```python
from build123d import *

# Parameters (mm, degrees)
EXTRUDE_1_DEPTH     = 25
EXTRUDE_2_DEPTH     = 2
CUT_EXTRUDE_1_DEPTH = 15
SKETCH_4_R          = 1.15
EXTRUDE_3_DEPTH     = 15
SKETCH_5_W          = 6.2
SKETCH_5_H          = 22
CUT_EXTRUDE_2_DEPTH = 74.581891949
SKETCH_6_W          = 6.2
SKETCH_6_H          = 2
CUT_EXTRUDE_3_DEPTH = 74.581891949
EXTRUDE_4_DEPTH     = 12
EXTRUDE_5_DEPTH     = 12


with BuildPart() as part:
    # 草图1 → 凸台-拉伸1 (new body)
    with BuildSketch(Plane.XY):
        Polygon((19.5, 14.714466094), (19.5, -3.035533906), (24.5, -3.035533906), (31.571067812, 4.035533906), (31.571067812, 41.75), (21.571067812, 51.75), (-21.571067812, 51.75), (-31.571067812, 41.75), (-31.571067812, 4.035533906), (-24.5, -3.035533906), (-19.5, -3.035533906), (-19.5, 14.714466094), (-26.571067812, 21.785533906), (-26.571067812, 36.75), (-21.571067812, 41.75), (21.571067812, 41.75), (26.571067812, 36.75), (26.571067812, 21.785533906), align=None)
    extrude(amount=EXTRUDE_1_DEPTH)

    # 草图2 → 凸台-拉伸2 (add)
    with BuildSketch(Plane.XY.offset(25)):
        Polygon((-26.571067812, 30.27081528), (-19.5, 23.199747468), (-19.5, 14.714466094), (-26.571067812, 21.785533906), align=None)
        Polygon((26.571067812, 30.27081528), (19.5, 23.199747468), (19.5, 14.714466094), (26.571067812, 21.785533906), align=None)
    extrude(amount=-EXTRUDE_2_DEPTH)

    # 草图3 → 切除-拉伸1 (cut)
    with BuildSketch(Plane(origin=(0, 0, 0), x_dir=(-1, 0, 0), z_dir=(0, 0, -1))):
        Polygon((26.571067812, 21.785533906), (24.5, -3.035533906), (31.571067812, 4.035533906), (31.571067812, 41.75), (21.571067812, 51.75), (-21.571067812, 51.75), (-31.571067812, 41.75), (-31.571067812, 4.035533906), (-24.5, -3.035533906), (-26.571067812, 21.785533906), (-26.571067812, 36.75), (-21.571067812, 41.75), (21.571067812, 41.75), (26.571067812, 36.75), align=None)
    extrude(amount=-CUT_EXTRUDE_1_DEPTH, mode=Mode.SUBTRACT)

    # 草图4 → 凸台-拉伸3 (add, symmetric)
    # profile 1 of 2: a face of its own
    with BuildSketch(Plane(origin=(0, 0, 0), x_dir=(0, 0, -1), z_dir=(1, 0, 0))):
        with BuildLine():
            Line((-12, 49.75), (-15, 49.75))
            ThreePointArc((-15, 49.75), (-18, 46.75), (-15, 43.75))
            Line((-15, 43.75), (-12, 43.75))
            ThreePointArc((-12, 43.75), (-9, 46.75), (-12, 49.75))
        make_face()
        with Locations((-12, 46.75)):
            Circle(SKETCH_4_R, mode=Mode.SUBTRACT)
    # profile 2 of 2: a face of its own
    with BuildSketch(Plane(origin=(0, 0, 0), x_dir=(0, 0, -1), z_dir=(1, 0, 0))):
        with BuildLine():
            Line((-14.716445048, 63.023156039), (-20, 51.75))
            Line((-20, 51.75), (-15, 51.75))
            Line((-15, 51.75), (-9.495412844, 60.098623853))
            ThreePointArc((-9.495412844, 60.098623853), (-10.533902095, 64.36735686), (-14.716445048, 63.023156039))
        make_face()
        with Locations((-12, 61.75)):
            Circle(SKETCH_4_R, mode=Mode.SUBTRACT)
    extrude(amount=EXTRUDE_3_DEPTH, both=True)

    # 草图5 → 切除-拉伸2 (cut, through all)
    with BuildSketch(Plane(origin=(0, 0, 15), x_dir=(-1, 0, 0), z_dir=(0, 0, -1))):
        with Locations((-6, 54.75)):
            Rectangle(SKETCH_5_W, SKETCH_5_H)
        with Locations((6, 54.75)):
            Rectangle(SKETCH_5_W, SKETCH_5_H)
    extrude(amount=CUT_EXTRUDE_2_DEPTH, mode=Mode.SUBTRACT)

    # 草图6 → 切除-拉伸3 (cut, through all)
    with BuildSketch(Plane(origin=(0, 0, 15), x_dir=(-1, 0, 0), z_dir=(0, 0, -1))):
        with Locations((-6, 61.418154436)):
            Rectangle(SKETCH_6_W, SKETCH_6_H)
        with Locations((6, 61.418154436)):
            Rectangle(SKETCH_6_W, SKETCH_6_H)
    extrude(amount=-CUT_EXTRUDE_3_DEPTH, mode=Mode.SUBTRACT)

    # 草图7 → 凸台-拉伸4 (add)
    with BuildSketch(Plane(origin=(0, 0, 0), x_dir=(-1, 0, 0), z_dir=(0, 0, -1))):
        Polygon((-26.571067812, 21.785533906), (-24.5, -3.035533906), (-19.5, -3.035533906), (-19.5, 14.714466094), align=None)
    extrude(amount=EXTRUDE_4_DEPTH)

    # 草图8 → 凸台-拉伸5 (add)
    with BuildSketch(Plane(origin=(0, 0, 0), x_dir=(-1, 0, 0), z_dir=(0, 0, -1))):
        Polygon((19.5, -3.035533906), (24.5, -3.035533906), (26.571067812, 21.785533906), (19.5, 14.714466094), align=None)
    extrude(amount=EXTRUDE_5_DEPTH)


solid = part.part
```
Build history of the part. All positions in model axes, mm. A direction names the side the tool comes from. Round coordinates to 2 decimals unless told otherwise and drop trailing zeros. Loops run counter-clockwise (first coordinate to the right, second up) from the corner with the lowest first, then second, coordinate; pieces in that order, holes last.
Item 1: Drill centre lines: line 1 along X through (y, z) = (32, 20); line 2 along Z through (x, y) = (0.15, 46.75); line 3 along Y through (x, z) = (-13.6, 12). Where is each one in solid material? Low to high.
Item 2: Saw through at A-A (y = 33). List the corners of the cut face in (x, z), then the cut area to 4 significant figures.
Item 3: Pin check, flat tips, straight feed: P1, Ø12, axis at x = -20, z = -8.5, coming from the +Y side; P2, Ø1.4, axis at y = 61.75, z = 12, coming from the +X side; P3, Ø7.5, axis at y = 57.5, z = 12, coming from the +X side; P4, Ø2.5, axis at x = -11.5, z = 13, coming from the -Y side. Stop position of each tip, or through.
Item 4: Which spindle directions (+Z, -Z, +X, -X, +Y, -Y) get a long thin tool onto all of the face, cutting with end or side? Do faces 1 (the face through (-24.106, 39.215, 19.93)), 2 (the face through (2.9, 46.7, 13.4)), 3 (the face through (25.55, 9.55, 1.69)). Say none if no direction does.
Item 5: Saw through at C-C (y = 46.75). List the corners of the cut face in (x, z).
Item 6: Two-plate mould, pull along Y, no slides. Class faces 4 (the face through (-15, 58, 15)), 5 (the face through (12, 43.75, 14)), 6 (the face through (22.986, 18.201, 5.745)): released by +Y, released by -Y, zero draft, split by the parting line, or undercut.
Item 7: Saw through at B-B (z = -9). List the corners of the cut face in (x, y), then the cut area to 3 significant figures.
Item 8: Saw through at D-D (y = 61.75). List the corners of the cut face in (x, z), then the cut area to 3 significant figures.
Worked answers:
1. line 1: x = -31.57 to -26.57, 26.57 to 31.57
1. line 2: z = 9 to 10.85, 13.15 to 25
1. line 3: y = 43.75 to 45.6, 47.9 to 49.75, 56.3 to 60.6, 62.9 to 64.75
2. outline: (-31.57, 15) - (-26.57, 15) - (-26.57, 25) - (-31.57, 25) - close; (26.57, 15) - (31.57, 15) - (31.57, 25) - (26.57, 25) - close
2. area: 100.0 mm2
3. P1: stops at y = 21.21
3. P2: passes through
3. P3: stops at x = 15
3. P4: stops at y = 43.75
4. face 1: +Z, -Z
4. face 2: -Z, +Y, -Y
4. face 3: -Z, +X, -Y
5. outline: (-26.57, 15) - (-15, 15) - (-15, 13.15) - (-9.1, 13.15) - (-9.1, 15) - (-2.9, 15) - (-2.9, 13.15) - (2.9, 13.15) - (2.9, 15) - (9.1, 15) - (9.1, 13.15) - (15, 13.15) - (15, 15) - (26.57, 15) - (26.57, 25) - (-26.57, 25) - close; (-15, 9) - (-9.1, 9) - (-9.1, 10.85) - (-15, 10.85) - close; (-2.9, 9) - (2.9, 9) - (2.9, 10.85) - (-2.9, 10.85) - close; (9.1, 9) - (15, 9) - (15, 10.85) - (9.1, 10.85) - close
6. face 4: zero draft
6. face 5: released by -Y
6. face 6: undercut
7. outline: (-26.57, 21.79) - (-24.5, -3.04) - (-19.5, -3.04) - (-19.5, 14.71) - close; (19.5, -3.04) - (24.5, -3.04) - (26.57, 21.79) - (19.5, 14.71) - close
7. area: 250 mm2
8. outline: (-15, 9) - (-9.1, 9) - (-9.1, 10.85) - (-15, 10.85) - close; (-15, 13.15) - (-9.1, 13.15) - (-9.1, 15.31) - (-15, 15.31) - close; (-2.9, 9) - (2.9, 9) - (2.9, 10.85) - (-2.9, 10.85) - close; (-2.9, 13.15) - (2.9, 13.15) - (2.9, 15.31) - (-2.9, 15.31) - close; (9.1, 9) - (15, 9) - (15, 10.85) - (9.1, 10.85) - close; (9.1, 13.15) - (15, 13.15) - (15, 15.31) - (9.1, 15.31) - close
8. area: 70.6 mm2
